Input: part model. Units: mm. Frame: model coordinates. Face numbers are marked on the shaded views. A direction names the side the tool comes from. Round coordinates to 2 decimals unless told otherwise and drop trailing zeros. Loops run counter-clockwise (first coordinate to the right, second up) from the corner with the lowest first, then second, coordinate; pieces in that order, holes last. Notation, with made-up numbers: (-7, 5.5) -> (45, 5.5) arc R22 ccw to (45, 14.5) -> close; hole circle Ø1 at (-36.75, -27.5). An arc over 180 degrees is marked (long way). Answer in a Markdown table with one row per item. Add a question column.
Q1. Reachability of the marked faces 5, 6 and 7 from +Z, -Z, +X, -X, +Y, -Y: full face, straight path, thin tool, end or side. Return the list, or none.
Q2. Ray query, L1, parallel to X at y = 1.5, z = -0.25; L2, parallel to X at y = 0, z = 2; L3, parallel to Z at x = -0.75, y = -1.5. Return the intervals inside material, ascending. Write a range as from..to.
Q3. Section D-D, the plane x = -7. Output: boundary loops of the cut face in (y, z) (3 decimals), and give its area (3 significant figures).
Q4. Mould query, pull axis Y, two halves, no side actions, for the marked faces 1, 2, 3 and 4. Classes: pulls with the +Y half, pulls with the -Y half, needs draft (parallel to the pull), parting line crosses it, or undercut.
Q5. Section C-C, the plane x = -4.75. Output: boundary loops of the cut face in (y, z), and give its area (3 significant figures).
Q6. Pin query (flat end, axial travel): pin 1 (1.2 mm diameter, centred on y = 1, z = 0, fed in from +X); pin 2 (2 mm diameter, centred on x = -5.5, z = 2, fed in from +Y); pin 3 (3 mm diameter, centred on x = -1, y = 4.5, fed in from +Z). Return the tip coordinate at first contact, or that it passes through.
Q7. Section A-A, the plane z = 0. Output: boundary loops of the cut face in (x, y).
Q8. Section B-B, the plane y = 0. Output: boundary loops of the cut face in (x, z), and give its area (3 significant figures).
```python
from build123d import *

# Parameters (mm, degrees)
ENL_V_MAT_EXTRU_1_DEPTH = 2


with BuildPart() as part:
    # Esquisse1 → R_volution1 (revolve)
    with BuildSketch(Plane.XY, mode=Mode.PRIVATE) as r_volution1_sk:
        with BuildLine():
            Line((0, 0), (0, 6))
            Line((0, 6), (-5.5, 6))
            Line((-5.5, 6), (-6, 5.25))
            Line((-6, 5.25), (-8, 5))
            Line((-8, 5), (-8, 3.624621125))
            ThreePointArc((-8, 3.624621125), (-7.83056435, 3.132291358), (-7.3940285, 2.848507125))
            Line((-7.3940285, 2.848507125), (-6.30298575, 2.575746437))
            ThreePointArc((-6.30298575, 2.575746437), (-6.084717825, 2.433854321), (-6, 2.187689437))
            Line((-6, 2.187689437), (-6, 0))
            Line((-6, 0), (0, 0))
        make_face()
    revolve(r_volution1_sk.sketch.rotate(Axis((3.088773822, 0, 0), (-1, 0, 0)), 90), axis=Axis((3.088773822, 0, 0), (-1, 0, 0)))

    # Esquisse2 → Enl_v. mat.-Extru.1 (cut)
    with BuildSketch(Plane(origin=(0, 0, 0), x_dir=(0, 0, -1), z_dir=(1, 0, 0))):
        with BuildLine():
            Line((-0.75, -1.5), (-0.75, 1.5))
            ThreePointArc((-0.75, 1.5), (0, 2.25), (0.75, 1.5))
            Line((0.75, 1.5), (0.75, -1.5))
            ThreePointArc((0.75, -1.5), (0, -2.25), (-0.75, -1.5))
        make_face()
    extrude(amount=-ENL_V_MAT_EXTRU_1_DEPTH, mode=Mode.SUBTRACT)


solid = part.part
```
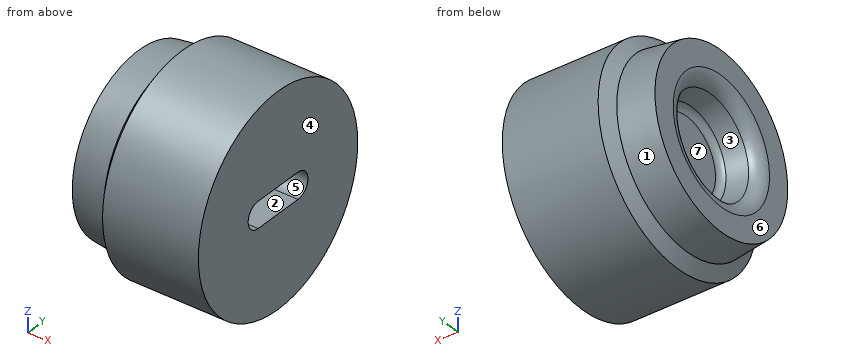
Answer block:
| question | item | result |
|---|---|---|
| 1 | face 5 | +X |
| 1 | face 6 | +Z, -Z, -X, +Y, -Y |
| 1 | face 7 | -X |
| 2 | L1 | -6..-2 |
| 2 | L2 | -6..0 |
| 2 | L3 | -5.81..-0.75, 0.75..5.81 |
| 3 | outline | circle Ø10.25 at (0, 0); hole circle Ø5.5 at (0, 0) |
| 3 | area | 58.8 mm^2 |
| 4 | face 1 | parting line crosses it |
| 4 | face 2 | undercut |
| 4 | face 3 | undercut |
| 4 | face 4 | needs draft |
| 5 | outline | circle Ø12 at (0, 0) |
| 5 | area | 113 mm^2 |
| 6 | pin 1 | x = -2 |
| 6 | pin 2 | y = 5.92 |
| 6 | pin 3 | z = 5.2 |
| 7 | outline | (-8, -5) -> (-6, -5.25) -> (-5.5, -6) -> (0, -6) -> (0, -2.25) -> (-2, -2.25) -> (-2, 2.25) -> (0, 2.25) -> (0, 6) -> (-5.5, 6) -> (-6, 5.25) -> (-8, 5) -> (-8, 3.62) arc R0.8 ccw to (-7.39, 2.85) -> (-6.3, 2.58) arc R0.4 cw to (-6, 2.19) -> (-6, -2.19) arc R0.4 cw to (-6.3, -2.58) -> (-7.39, -2.85) arc R0.8 ccw to (-8, -3.62) -> close |
| 8 | outline | (-8, -5) -> (-6, -5.25) -> (-5.5, -6) -> (0, -6) -> (0, -0.75) -> (-2, -0.75) -> (-2, 0.75) -> (0, 0.75) -> (0, 6) -> (-5.5, 6) -> (-6, 5.25) -> (-8, 5) -> (-8, 3.62) arc R0.8 ccw to (-7.39, 2.85) -> (-6.3, 2.58) arc R0.4 cw to (-6, 2.19) -> (-6, -2.19) arc R0.4 cw to (-6.3, -2.58) -> (-7.39, -2.85) arc R0.8 ccw to (-8, -3.62) -> close |
| 8 | area | 78.0 mm^2 |
